```python
from build123d import *

# Parameters (mm, degrees)
SKETCH1_W           = 1
SKETCH1_H           = 1
SKETCH1_W_2         = 6
SKETCH1_H_2         = 6
SKETCH1_R           = 2.1
BOSS_EXTRUDE1_DEPTH = 50.8
FILLET1_R           = 1


with BuildPart() as part:
    # Sketch1 → Boss-Extrude1 (new body)
    # profile 1 of 35: a face of its own
    with BuildSketch(Plane.XY):
        Polygon((-6, 7), (-6, 8), (-7, 8), align=None)
    # profile 2 of 35: a face of its own
    with BuildSketch(Plane.XY):
        Polygon((-6, 7), (-7, 8), (-8, 8), (-8, 7), (-7, 6), (-6, 6), align=None)
    # profile 3 of 35: a face of its own
    with BuildSketch(Plane.XY):
        Polygon((-8, 7), (-8, 6), (-7, 6), align=None)
    # profile 4 of 35: a face of its own
    with BuildSketch(Plane.XY):
        Polygon((-3, 8), (-3, 10), (-10, 10), (-10, 3), (-8, 3), (-8, 6), (-8, 7), (-8, 8), (-7, 8), (-6, 8), align=None)
    # profile 5 of 35: a face of its own
    with BuildSketch(Plane.XY):
        Polygon((-6, 5), (-6, 6), (-7, 6), align=None)
    # profile 6 of 35: a face of its own
    with BuildSketch(Plane.XY):
        Polygon((-6, 6), (-5, 6), (-6, 7), align=None)
    # profile 7 of 35: a face of its own
    with BuildSketch(Plane.XY):
        Polygon((-3, 4), (-5, 6), (-6, 6), (-6, 5), (-4, 3), (-4, 4), align=None)
    # profile 8 of 35: a face of its own
    with BuildSketch(Plane.XY):
        with Locations((-3.5, 3.5)):
            Rectangle(SKETCH1_W, SKETCH1_H)
    # profile 9 of 35: a face of its own
    with BuildSketch(Plane.XY):
        with Locations((0, 3.5)):
            Rectangle(SKETCH1_W_2, SKETCH1_H)
    # profile 10 of 35: a face of its own
    with BuildSketch(Plane.XY):
        with Locations((-3.5, 0)):
            Rectangle(SKETCH1_W, SKETCH1_H_2)
    # profile 11 of 35: a face of its own
    with BuildSketch(Plane.XY):
        Rectangle(SKETCH1_W_2, SKETCH1_H_2)
        Circle(SKETCH1_R, mode=Mode.SUBTRACT)
    # profile 12 of 35: a face of its own
    with BuildSketch(Plane.XY):
        with Locations((3.5, 3.5)):
            Rectangle(SKETCH1_W, SKETCH1_H)
    # profile 13 of 35: a face of its own
    with BuildSketch(Plane.XY):
        Polygon((6, 6), (5, 6), (3, 4), (4, 4), (4, 3), (6, 5), align=None)
    # profile 14 of 35: a face of its own
    with BuildSketch(Plane.XY):
        Polygon((6, 7), (5, 6), (6, 6), align=None)
    # profile 15 of 35: a face of its own
    with BuildSketch(Plane.XY):
        Polygon((6, 6), (6, 5), (7, 6), align=None)
    # profile 16 of 35: a face of its own
    with BuildSketch(Plane.XY):
        Polygon((8, 8), (7, 8), (6, 7), (6, 6), (7, 6), (8, 7), align=None)
    # profile 17 of 35: a face of its own
    with BuildSketch(Plane.XY):
        Polygon((7, 8), (6, 8), (6, 7), align=None)
    # profile 18 of 35: a face of its own
    with BuildSketch(Plane.XY):
        Polygon((7, 6), (8, 6), (8, 7), align=None)
    # profile 19 of 35: a face of its own
    with BuildSketch(Plane.XY):
        Polygon((10, 3), (10, 10), (3, 10), (3, 8), (6, 8), (7, 8), (8, 8), (8, 7), (8, 6), (8, 3), align=None)
    # profile 20 of 35: a face of its own
    with BuildSketch(Plane.XY):
        with Locations((3.5, 0)):
            Rectangle(SKETCH1_W, SKETCH1_H_2)
    # profile 21 of 35: a face of its own
    with BuildSketch(Plane.XY):
        with Locations((3.5, -3.5)):
            Rectangle(SKETCH1_W, SKETCH1_H)
    # profile 22 of 35: a face of its own
    with BuildSketch(Plane.XY):
        Polygon((6, -6), (6, -5), (4, -3), (4, -4), (3, -4), (5, -6), align=None)
    # profile 23 of 35: a face of its own
    with BuildSketch(Plane.XY):
        Polygon((7, -6), (6, -5), (6, -6), align=None)
    # profile 24 of 35: a face of its own
    with BuildSketch(Plane.XY):
        Polygon((6, -7), (6, -6), (5, -6), align=None)
    # profile 25 of 35: a face of its own
    with BuildSketch(Plane.XY):
        Polygon((8, -8), (8, -7), (7, -6), (6, -6), (6, -7), (7, -8), align=None)
    # profile 26 of 35: a face of its own
    with BuildSketch(Plane.XY):
        Polygon((6, -7), (6, -8), (7, -8), align=None)
    # profile 27 of 35: a face of its own
    with BuildSketch(Plane.XY):
        Polygon((8, -7), (8, -6), (7, -6), align=None)
    # profile 28 of 35: a face of its own
    with BuildSketch(Plane.XY):
        Polygon((10, -10), (10, -3), (8, -3), (8, -6), (8, -7), (8, -8), (7, -8), (6, -8), (3, -8), (3, -10), align=None)
    # profile 29 of 35: a face of its own
    with BuildSketch(Plane.XY):
        with Locations((0, -3.5)):
            Rectangle(SKETCH1_W_2, SKETCH1_H)
    # profile 30 of 35: a face of its own
    with BuildSketch(Plane.XY):
        with Locations((-3.5, -3.5)):
            Rectangle(SKETCH1_W, SKETCH1_H)
    # profile 31 of 35: a face of its own
    with BuildSketch(Plane.XY):
        Polygon((-4, -3), (-6, -5), (-6, -6), (-5, -6), (-3, -4), (-4, -4), align=None)
    # profile 32 of 35: a face of its own
    with BuildSketch(Plane.XY):
        Polygon((-6, -7), (-5, -6), (-6, -6), align=None)
    # profile 33 of 35: a face of its own
    with BuildSketch(Plane.XY):
        Polygon((-6, -6), (-6, -5), (-7, -6), align=None)
    # profile 34 of 35: a face of its own
    with BuildSketch(Plane.XY):
        Polygon((-7, -6), (-8, -7), (-8, -8), (-7, -8), (-6, -7), (-6, -6), align=None)
    # profile 35 of 35: a face of its own
    with BuildSketch(Plane.XY):
        Polygon((-8, -3), (-10, -3), (-10, -10), (-3, -10), (-3, -8), (-6, -8), (-7, -8), (-8, -8), (-8, -7), (-8, -6), align=None)
    extrude(amount=BOSS_EXTRUDE1_DEPTH)

    # Fillet1
    fillet1_edges = [part.edges().sort_by_distance(p)[0] for p in [
        (-10, -10, 25.4),
        (-10, 10, 25.4),
        (10, 10, 25.4),
        (10, -10, 25.4),
    ]]
    fillet(fillet1_edges, radius=FILLET1_R)


solid = part.part
```
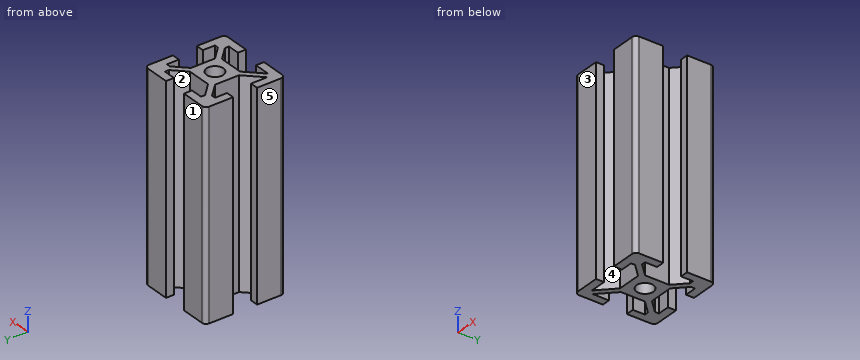
Source: CAD feature listing. Evaluate the final solid. Frame: model axes, mm. Face numbers are marked on the shaded views. A direction names the side the tool comes from. Coordinates: 2 decimals unless noted, no trailing zeros. Loops run counter-clockwise (first coordinate to the right, second up) from the corner with the lowest first, then second, coordinate; pieces in that order, holes last. Notation, with made-up numbers: M -33.5,-23.75 L 17.5,-23.75 A15 cw 17.5,-6.75 Z; hole C 31.25,56 d2. An arc over 180 degrees is marked long. Use CSV: the item, a comma, the result in double quotes.
(1) Cut plane B-B on y = 0. Return loops of the section in (x, z), and give its area (3 significant figures).
Answers follow:
outline,"M -4,0 L -2.1,0 L -2.1,50.8 L -4,50.8 Z; M 2.1,0 L 4,0 L 4,50.8 L 2.1,50.8 Z"
area,"193 mm²"
(2) Cut plane D-D on y = 3.5. Return loops of the section in (x, z), and give its area (3 significant figures).
Answers follow:
outline,"M -10,0 L -8,0 L -8,50.8 L -10,50.8 Z; M -4.5,0 L 4.5,0 L 4.5,50.8 L -4.5,50.8 Z; M 8,0 L 10,0 L 10,50.8 L 8,50.8 Z"
area,"660 mm²"
(3) Cut plane A-A on x = -4.5. Return loops of the section in (y, z).
Answers follow:
outline,"M -10,0 L -8,0 L -8,50.8 L -10,50.8 Z; M -5.5,0 L -3.5,0 L -3.5,50.8 L -5.5,50.8 Z; M 3.5,0 L 5.5,0 L 5.5,50.8 L 3.5,50.8 Z; M 8,0 L 10,0 L 10,50.8 L 8,50.8 Z"
(4) Draft query along Y for the marked faces 3, 4 and 5. Return one class per face: pulls with the +Y half, pulls with the -Y half, needs draft (parallel to the pull), parting line crosses it, or undercut.
Answers follow:
face 3,"pulls with the -Y half"
face 4,"undercut"
face 5,"needs draft"
(5) Reachability of the marked faces 1 and 2 from +Z, -Z, +X, -X, +Y, -Y: full face, straight path, thin tool, end or side. Return the list, or none.
Answers follow:
face 1,"+Z, -Z, +X, -X, +Y"
face 2,"+Z, -Z"
(6) Line query: line 1 (X direction, y = 9, z = 22); line 2 (Y direction, x = -3.25, z = 6); line 3 (X direction, y = -5.25, z = 8.5). Output: solid intervals per line, ascending. Write a range as [from, to].
Answers follow:
line 1,"[-10, -3], [3, 10]"
line 2,"[-10, -8], [-4.25, 4.25], [8, 10]"
line 3,"[-10, -8], [-6.25, -4.25], [4.25, 6.25], [8, 10]"
(7) Contact query for flat-ended pins moving along their axis: pin 1 (0.6 mm diameter, centred on y = 9.5, z = 13, fed in from +X); pin 2 (12 mm diameter, centred on x = -2.5, y = 5, fed in from -Z); pin 3 (3 mm diameter, centred on x = 0.5, z = 24, fed in from +Y). Output: stop coordinate, or through.
Answers follow:
pin 1,"x = 9.98"
pin 2,"z = 0"
pin 3,"y = 4"
